```python
from build123d import *

# Parameters (mm, degrees)
SKETCH_1_W               = 16.3
SKETCH_1_H               = 3
SKETCH_1_W_2             = 5
SKETCH_1_H_2             = 16
SKETCH_19_W              = 3
SKETCH_19_H              = 0.05
EXTRUDE_START            = 14
SKETCH_20_R              = 18
EXTRUDE_2_DEPTH          = 14
CUT_EXTRUDE_6_DEPTH      = 3
CUT_EXTRUDE_4_DEPTH      = 12
SKETCH_13_R              = 1.5
CUT_EXTRUDE_8_DEPTH      = 7
PATTERN_CIRCULAR_2_COUNT = 4
FILLET_1_R               = 0.5
SKETCH_21_R              = 20
CUT_EXTRUDE_7_DEPTH      = 42.3


with BuildPart() as part:
    # Эскиз1 → Повернуть1 основной корпус (revolve)
    with BuildSketch(Plane(origin=(0, 0, 0), x_dir=(1, 0, 0), z_dir=(0, 1, 0)), mode=Mode.PRIVATE) as revolve_1_sk:
        with Locations((8.15, 1.5)):
            Rectangle(SKETCH_1_W, SKETCH_1_H)
        Polygon((16.3, 0), (19.3, 0), (19.3, 10), (16.3, 10), (16.3, 3), align=None)
        Polygon((24.3, 0), (24.3, 16), (20.3, 16), (19.3, 15), (19.3, 10), (19.3, 0), align=None)
        Polygon((40.8, 17.5), (42.3, 16), (42.3, 0), (24.3, 0), (24.3, 16), (25.8, 17.5), align=None)
        with Locations((44.8, 8)):
            Rectangle(SKETCH_1_W_2, SKETCH_1_H_2)
        with BuildLine():
            ThreePointArc((47.3, 16), (47.885786438, 17.414213562), (49.3, 18))
            Line((49.3, 18), (104.3, 18))
            Line((104.3, 18), (104.3, 0))
            Line((104.3, 0), (47.3, 0))
            Line((47.3, 0), (47.3, 16))
        make_face()
    revolve(revolve_1_sk.sketch.rotate(Axis((0, 0, 0), (1, 0, 0)), 180), axis=Axis((0, 0, 0), (1, 0, 0)))

    # Эскиз19 → Вырез-Повернуть2 пластиковая часть (revolve, cut)
    with BuildSketch(Plane(origin=(0, 0, 0), x_dir=(1, 0, 0), z_dir=(0, 1, 0)), mode=Mode.PRIVATE) as cut_revolve_2_sk:
        with Locations((102.8, 17.975)):
            Rectangle(SKETCH_19_W, SKETCH_19_H)
    revolve(cut_revolve_2_sk.sketch.rotate(Axis((103.004702911, 0, 0), (-1, 0, 0)), 180), axis=Axis((103.004702911, 0, 0), (-1, 0, 0)), mode=Mode.SUBTRACT)

    # Эскиз20 → Бобышка-Вытянуть2 пластиковая крышка контактов (add)
    with BuildSketch(Plane(origin=(104.3, 0, 0), x_dir=(0, 0, -1), z_dir=(1, 0, 0)).offset(EXTRUDE_START)):
        with Locations(Location((0, 0, 0), (0, 0, 180))):
            Circle(SKETCH_20_R)
    extrude(amount=-EXTRUDE_2_DEPTH)

    # Эскиз11 → Вырез-Вытянуть6 (cut)
    with BuildSketch(Plane.ZY.offset(-16.3)):
        with BuildLine():
            ThreePointArc((4.358898944, 9), (0, 10), (-4.358898944, 9))
            Line((-4.358898944, 9), (4.358898944, 9))
        make_face()
        with BuildLine():
            Line((4.358898944, -9), (-4.358898944, -9))
            ThreePointArc((-4.358898944, -9), (0, -10), (4.358898944, -9))
        make_face()
    extrude(amount=-CUT_EXTRUDE_6_DEPTH, mode=Mode.SUBTRACT)

    # Эскиз6 → Вырез-Вытянуть4 на оси (cut)
    with BuildSketch(Plane.ZY):
        with BuildLine():
            Line((-1.75306936, 2.434491286), (1.561110291, 2.561822527))
            ThreePointArc((1.561110291, 2.561822527), (-0.115175441, 2.997788288), (-1.75306936, 2.434491286))
        make_face()
    extrude(amount=-CUT_EXTRUDE_4_DEPTH, mode=Mode.SUBTRACT)

    # Эскиз13 → Вырез-Вытянуть8 для винтов (cut)
    with BuildSketch(Plane.ZY.offset(-19.3)):
        with Locations((-9.192388155, 9.192388155)):
            Circle(SKETCH_13_R)
    cut_extrude_8 = extrude(amount=-CUT_EXTRUDE_8_DEPTH, mode=Mode.SUBTRACT)

    # Круговой массив2 для винтов: Вырез-Вытянуть8 для винтов ×4 about axis
    pattern_circular_2_axis = Axis((0, 0, 0), (1, 0, 0))
    for i in range(1, PATTERN_CIRCULAR_2_COUNT):
        add(cut_extrude_8.rotate(pattern_circular_2_axis, i * 360 / PATTERN_CIRCULAR_2_COUNT), mode=Mode.SUBTRACT)

    # Скругление1
    # the kernel refuses this fillet: 0.5 mm, written as the material it takes off along each edge
    with BuildSketch(Plane(origin=(19.3, 0, 0), x_dir=(0, 0, 1), z_dir=(0, 1, 0))) as fillet_1_piece_1:
        with BuildLine():
            CenterArc((15 - FILLET_1_R * 0.414213562373, FILLET_1_R), FILLET_1_R, 270, 45)
            Line((15 - FILLET_1_R * 0.414213562373, 0), (15, 0))
            Line((15, 0), (15 + FILLET_1_R * 0.292893218813, FILLET_1_R * 0.292893218813))
        make_face()
    revolve(axis=Axis((19.3, 0, 0), (1, 0, 0)), mode=Mode.SUBTRACT)
    with BuildSketch(Plane(origin=(118.3, 0, 0), x_dir=(0, 0, 1), z_dir=(0, 1, 0))) as fillet_1_piece_2:
        with BuildLine():
            CenterArc((18 - FILLET_1_R, -FILLET_1_R), FILLET_1_R, 0, 90)
            Line((18 - FILLET_1_R, 0), (18, 0))
            Line((18, 0), (18, -FILLET_1_R))
        make_face()
    revolve(axis=Axis((118.3, 0, 0), (1, 0, 0)), mode=Mode.SUBTRACT)
    with BuildSketch(Plane(origin=(16.001803864, 9, -4.358898944), x_dir=(0, 0, 1), z_dir=(1, 0, 0))) as fillet_1_piece_3:
        with BuildLine():
            CenterArc((0.116258256, 0.5), FILLET_1_R, 243.474647983, 26.525352017)
            ThreePointArc((-0.107038622, 0.052631579), (-0.053597784, 0.026156196), (0, 0))
            Line((0, 0), (0.116258256, 0))
        make_face()
    extrude(amount=3.298196136, mode=Mode.SUBTRACT)
    with BuildSketch(Plane(origin=(16.001803864, 9, 4.358898944), x_dir=(0, -0.4412496727830022, 0.8973843804462464), z_dir=(1, 0, 0))) as fillet_1_piece_4:
        with BuildLine():
            CenterArc((0.116296493, 0.499991108), FILLET_1_R, 243.81635761, 26.525352017)
            Line((-0.104328343, 0.051298918), (0, 0))
            ThreePointArc((0, 0), (0.059639227, -0.000177843), (0.119278454, 0))
        make_face()
    extrude(amount=3.298196136, mode=Mode.SUBTRACT)
    with BuildSketch(Plane(origin=(16.3, 9, -5.608898944), x_dir=(1, 0, 0), z_dir=(0, 0, 1)), Plane(origin=(16.3, -9, 5.608898944), x_dir=(1, 0, 0), z_dir=(0, 0, -1))) as fillet_1_piece_5:
        with BuildLine():
            CenterArc((FILLET_1_R, -FILLET_1_R), FILLET_1_R, 90, 90)
            Line((0, -FILLET_1_R), (0, 0))
            Line((0, 0), (FILLET_1_R, 0))
        make_face()
    extrude(amount=11.217797887, mode=Mode.SUBTRACT)
    with BuildSketch(Plane(origin=(16.001803864, -9, 4.358898944), x_dir=(0, 0.4412496727830018, 0.8973843804462466), z_dir=(1, 0, 0))) as fillet_1_piece_6:
        with BuildLine():
            CenterArc((0.116296493, -0.499991108), FILLET_1_R, 89.658290373, 26.525352017)
            Line((-0.104328343, -0.051298918), (0, 0))
            ThreePointArc((0, 0), (0.059639227, 0.000177843), (0.119278454, 0))
        make_face()
    extrude(amount=3.298196136, mode=Mode.SUBTRACT)
    with BuildSketch(Plane(origin=(16.001803864, -9, -4.358898944), x_dir=(0, 0, 1), z_dir=(1, 0, 0))) as fillet_1_piece_7:
        with BuildLine():
            CenterArc((0.116258256, -0.5), FILLET_1_R, 90, 26.525352017)
            ThreePointArc((-0.107038622, -0.052631579), (-0.053597784, -0.026156196), (0, 0))
            Line((0, 0), (0.116258256, 0))
        make_face()
    extrude(amount=3.298196136, mode=Mode.SUBTRACT)
    with BuildSketch(Plane(origin=(19.3, 9.192388155, -9.192388155), x_dir=(0, 0, 1), z_dir=(0, -1, 0))) as fillet_1_piece_8:
        with BuildLine():
            CenterArc((1.5 + FILLET_1_R, -FILLET_1_R), FILLET_1_R, 90, 90)
            Line((1.5, -FILLET_1_R), (1.5, 0))
            Line((1.5, 0), (1.5 + FILLET_1_R, 0))
        make_face()
    revolve(axis=Axis((19.3, 9.192388155, -9.192388155), (-1, 0, 0)), mode=Mode.SUBTRACT)
    with BuildSketch(Plane(origin=(19.3, -9.192388155, -9.192388155), x_dir=(0, 1, 0), z_dir=(0, 0, 1))) as fillet_1_piece_9:
        with BuildLine():
            CenterArc((1.5 + FILLET_1_R, -FILLET_1_R), FILLET_1_R, 90, 90)
            Line((1.5, -FILLET_1_R), (1.5, 0))
            Line((1.5, 0), (1.5 + FILLET_1_R, 0))
        make_face()
    revolve(axis=Axis((19.3, -9.192388155, -9.192388155), (-1, 0, 0)), mode=Mode.SUBTRACT)
    with BuildSketch(Plane(origin=(19.3, -9.192388155, 9.192388155), x_dir=(0, 0, -1), z_dir=(0, 1, 0))) as fillet_1_piece_10:
        with BuildLine():
            CenterArc((1.5 + FILLET_1_R, -FILLET_1_R), FILLET_1_R, 90, 90)
            Line((1.5, -FILLET_1_R), (1.5, 0))
            Line((1.5, 0), (1.5 + FILLET_1_R, 0))
        make_face()
    revolve(axis=Axis((19.3, -9.192388155, 9.192388155), (-1, 0, 0)), mode=Mode.SUBTRACT)
    with BuildSketch(Plane(origin=(19.3, 9.192388155, 9.192388155), x_dir=(0, -1, 0), z_dir=(0, 0, -1))) as fillet_1_piece_11:
        with BuildLine():
            CenterArc((1.5 + FILLET_1_R, -FILLET_1_R), FILLET_1_R, 90, 90)
            Line((1.5, -FILLET_1_R), (1.5, 0))
            Line((1.5, 0), (1.5 + FILLET_1_R, 0))
        make_face()
    revolve(axis=Axis((19.3, 9.192388155, 9.192388155), (-1, 0, 0)), mode=Mode.SUBTRACT)
    # the kernel refuses this fillet: 0.5 mm, written as the material it adds along each edge
    with BuildSketch(Plane(origin=(19.3, 0, 0), x_dir=(0, -0.8947368421052432, -0.4465937565389121), z_dir=(0, -0.4465937565389121, 0.8947368421052432))) as fillet_1_2_piece_1:
        with BuildLine():
            CenterArc((10 + FILLET_1_R, -FILLET_1_R), FILLET_1_R, 90, 90)
            Line((10, -FILLET_1_R), (10, 0))
            Line((10, 0), (10 + FILLET_1_R, 0))
        make_face()
    revolve(axis=Axis((19.3, 0, 0), (1, 0, 0)), revolution_arc=126.949295967)
    with BuildSketch(Plane(origin=(19.3, 9, -4.242640687), x_dir=(0, 1, 0), z_dir=(0, 0, 1)), Plane(origin=(19.3, -9, 4.242640687), x_dir=(0, -1, 0), z_dir=(0, 0, -1))) as fillet_1_2_piece_2:
        with BuildLine():
            CenterArc((FILLET_1_R, FILLET_1_R), FILLET_1_R, 180, 90)
            Line((0, FILLET_1_R), (0, 0))
            Line((0, 0), (FILLET_1_R, 0))
        make_face()
    extrude(amount=8.485281374)
    with BuildSketch(Plane(origin=(19.3, 0, 0), x_dir=(0, 0.894736842105243, 0.44659375653891253), z_dir=(0, 0.44659375653891253, -0.894736842105243))) as fillet_1_2_piece_3:
        with BuildLine():
            CenterArc((10 + FILLET_1_R, -FILLET_1_R), FILLET_1_R, 90, 90)
            Line((10, -FILLET_1_R), (10, 0))
            Line((10, 0), (10 + FILLET_1_R, 0))
        make_face()
    revolve(axis=Axis((19.3, 0, 0), (1, 0, 0)), revolution_arc=126.949295967)
    with BuildSketch(Plane(origin=(19.3, -8.5, 4.242640687), x_dir=(0, -0.8947368421052433, 0.446593756538912), z_dir=(0, 0.446593756538912, 0.8947368421052433))) as fillet_1_2_piece_4:
        with BuildLine():
            CenterArc((0.5 + FILLET_1_R, -FILLET_1_R), FILLET_1_R, 90, 90)
            Line((0.5, -FILLET_1_R), (0.5, 0))
            Line((0.5, 0), (0.5 + FILLET_1_R, 0))
        make_face()
    revolve(axis=Axis((19.3, -8.5, 4.242640687), (1, 0, 0)), revolution_arc=26.525352017)
    with BuildSketch(Plane(origin=(19.3, -8.5, -4.242640687), x_dir=(0, -1, 0), z_dir=(0, 0, 1))) as fillet_1_2_piece_5:
        with BuildLine():
            CenterArc((0.5 + FILLET_1_R, -FILLET_1_R), FILLET_1_R, 90, 90)
            Line((0.5, -FILLET_1_R), (0.5, 0))
            Line((0.5, 0), (0.5 + FILLET_1_R, 0))
        make_face()
    revolve(axis=Axis((19.3, -8.5, -4.242640687), (1, 0, 0)), revolution_arc=26.525352017)
    with BuildSketch(Plane(origin=(19.3, 8.5, 4.242640687), x_dir=(0, 0.8947368421052433, 0.446593756538912), z_dir=(0, -0.446593756538912, 0.8947368421052433))) as fillet_1_2_piece_6:
        with BuildLine():
            CenterArc((0.5 + FILLET_1_R, FILLET_1_R), FILLET_1_R, 180, 90)
            Line((0.5, FILLET_1_R), (0.5, 0))
            Line((0.5, 0), (0.5 + FILLET_1_R, 0))
        make_face()
    revolve(axis=Axis((19.3, 8.5, 4.242640687), (-1, 0, 0)), revolution_arc=26.525352017)
    with BuildSketch(Plane(origin=(19.3, 8.5, -4.242640687), x_dir=(0, 1, 0), z_dir=(0, 0, 1))) as fillet_1_2_piece_7:
        with BuildLine():
            CenterArc((0.5 + FILLET_1_R, FILLET_1_R), FILLET_1_R, 180, 90)
            Line((0.5, FILLET_1_R), (0.5, 0))
            Line((0.5, 0), (0.5 + FILLET_1_R, 0))
        make_face()
    revolve(axis=Axis((19.3, 8.5, -4.242640687), (-1, 0, 0)), revolution_arc=26.525352017)

    # Эскиз21 → Вырез-Вытянуть7 (cut)
    with BuildSketch(Plane.ZY):
        Circle(SKETCH_21_R)
    extrude(amount=-CUT_EXTRUDE_7_DEPTH, mode=Mode.SUBTRACT)


solid = part.part
```
Geometry: final body of the model. Coordinates: model frame, mm. A direction names the side the tool comes from. Coordinates: 2 decimals unless noted, no trailing zeros. Order: outer loops, then holes, each group sorted by start corner. A loop starts at its lowest first (then second) coordinate and runs counter-clockwise, first axis right, second up. Notation, with made-up numbers: M 87.5,-12.5 L 145.5,-12.5 A28 ccw 145.5,11.5 Z; hole C -17.75,25 d8. An arc over 180 degrees is marked long. Answer in a Markdown table with one row per item. Add a question column.
Q1. Reachability of faces 1 (the cylindrical face through (44.83, 15.62, -3.47)), 2 (the cylindrical face through (75.664, -12.165, -13.267)) from +Z, -Z, +X, -X, +Y, -Y: full face, straight path, thin tool, end or side. Return the list, or none.
Q2. Section query A-A on x = 67.5. Return the cut outline in (y, z).
Q3. Section query B-B on x = 48.5. Return the cut outline in (y, z), and give its area (3 significant figures).
Q4. Line query: L1, parallel to Z at x = 78.5, y = -1.5; L2, parallel to Y at x = 91.5, z = 4; L3, parallel to Y at x = 47, z = 0.5. Output: solid intervals per line, ascending.
Q5. Contact query for flat-ended pins moving along their axis: P1, Ø1.5, axis at x = 76, y = -1.5, coming from the -Z side; P2, Ø4, axis at x = 70, z = 9, coming from the +Y side; P3, Ø3, axis at x = 77, y = 11.5, coming from the +Z side. Output: stop coordinate, or through.
Completed:
| question | item | result |
|---|---|---|
| 1 | face 1 | -X |
| 1 | face 2 | +X, -X |
| 2 | outline | C 0,0 d36 |
| 3 | outline | C 0,0 d35.67 |
| 3 | area | 999 mm2 |
| 4 | L1 | z = -17.94 to 17.94 |
| 4 | L2 | y = -17.55 to 17.55 |
| 4 | L3 | y = -15.99 to 15.99 |
| 5 | P1 | stops at z = -17.98 |
| 5 | P2 | stops at y = 16.58 |
| 5 | P3 | stops at z = 14.97 |
